```python
from build123d import *

# Parameters (mm, degrees)
F1_DEPTH = 50
F2_R     = 5
F3_DEPTH = 25
F4_R     = 5
F5_DEPTH = 25


with BuildPart() as f1:
    # F0 (on Front) → F1 (new body)
    with BuildSketch(Plane.XZ):
        with BuildLine():
            ThreePointArc((-43.8768457623, 71.994107108), (-55.1426401019, 67.2817681029), (-59.8027732582, 55.9942785694))
            Line((-59.8027732582, 55.9942785694), (-59.8027732582, -8.5240794845))
            Line((-59.8027732582, -8.5240794845), (-53.8027732582, -8.5240794845))
            Line((-53.8027732582, -8.5240794845), (-53.8027732582, 56.4759205155))
            ThreePointArc((-53.8027732582, 56.4759205155), (-50.8738410701, 63.5469883274), (-43.8027732582, 66.4759205155))
            Line((-43.8027732582, 66.4759205155), (60.1959407812, 66.4759205155))
            Line((60.1959407812, 66.4759205155), (60.1959407812, 72.4759205155))
            Line((60.1959407812, 72.4759205155), (-43.8768457623, 71.994107108))
        make_face()
    extrude(amount=F1_DEPTH)

    # F2 (on face) → F3 (cut)
    with BuildSketch(Plane(origin=(-0.3342358086, 0, 72.1956911529), x_dir=(0.9999892837, 0, 0.0046295315), z_dir=(-0.0046295315, 0, 0.9999892837))):
        with Locations((-29.4691747415, -25)):
            Circle(F2_R)
        with Locations((30.5308252585, -25)):
            Circle(F2_R)
    extrude(amount=-F3_DEPTH, mode=Mode.SUBTRACT)

    # F4 (on face) → F5 (cut)
    with BuildSketch(Plane.YZ.offset(-53.8027732582)):
        with Locations((-12.5, 6.4759205155)):
            Circle(F4_R)
        with Locations((-37.5, 26.4759205155)):
            Circle(F4_R)
    extrude(amount=-F5_DEPTH, mode=Mode.SUBTRACT)


solid = f1.part
```
CAD build for the part. Positions are in the model's coordinates, mm. Give positions to 0.01 mm unless a question says otherwise; leave off trailing zeros. Order: outer loops, then holes, each group sorted by start corner. A loop starts at its lowest first (then second) coordinate and runs counter-clockwise, first axis right, second up.
(1) Drill centre lines: L1, parallel to X at y = -47, z = 5; L2, parallel to Z at x = -20.5, y = -29; L3, parallel to Z at x = -57, y = -12. Where is each one in solid material? Low to high.
(2) Saw through at A-A, the plane y = -37.5. Give the cut face in (x, z), then the cut area to 3 significant figures.
(3) Flat gauge pins, fed straight in: pin 1 (8 mm diameter, centred on y = -20, z = 10.5, fed in from +X); pin 2 (4 mm diameter, centred on x = -12.5, y = -23, fed in from -Z); pin 3 (1 mm diameter, centred on x = 46, y = -26, fed in from +Z); pin 4 (8 mm diameter, centred on y = -12.5, z = 6.48, fed in from +X). Where does each tip first touch, or does it go through?
(4) Saw through at D-D, the plane x = -48.5. Give the cut face in (y, z).
(5) Saw through at B-B, the plane z = 9. Give the cut face in (x, y).
(6) Mould opens along Z. For faces 1 (the flat face through (-53.803, -25, 24)), 2 (the cylindrical face through (-55.018, -24.65, 67.405)), 3 (the cylindrical face through (-56.76, -7.73, 7.98)) say: released by +Z, released by -Z, zero draft, split by the parting line, or undercut.
(7) Saw through at C-C, the plane y = -13.5. Give the cut face in (x, z).
Results found:
1. L1: x = -59.8 to -53.8
1. L2: z = 66.48 to 72.1
1. L3: z = -8.52 to 1.5, 11.45 to 65.04
2. outline: (-59.8, -8.52) - (-53.8, -8.52) - (-53.8, 21.48) - (-59.8, 21.48) - close; (-59.8, 31.48) - (-53.8, 31.48) - (-53.8, 56.48) arc R10 cw to (-43.8, 66.48) - (60.2, 66.48) - (60.2, 72.48) - (-43.88, 71.99) arc R16 ccw to (-59.8, 55.99) - close
2. area: 1,040 mm2
3. pin 1: stops at x = -53.8
3. pin 2: stops at z = 66.48
3. pin 3: stops at z = 72.41
3. pin 4: passes through
4. outline: (-50, 65.3) - (0, 65.3) - (0, 71.29) - (-50, 71.29) - close
5. outline: (-59.8, -50) - (-53.8, -50) - (-53.8, -16.82) - (-59.8, -16.82) - close; (-59.8, -8.18) - (-53.8, -8.18) - (-53.8, 0) - (-59.8, 0) - close
6. face 1: zero draft
6. face 2: released by +Z
6. face 3: undercut
7. outline: (-59.8, -8.52) - (-53.8, -8.52) - (-53.8, 1.58) - (-59.8, 1.58) - close; (-59.8, 11.37) - (-53.8, 11.37) - (-53.8, 56.48) arc R10 cw to (-43.8, 66.48) - (60.2, 66.48) - (60.2, 72.48) - (-43.88, 71.99) arc R16 ccw to (-59.8, 55.99) - close
